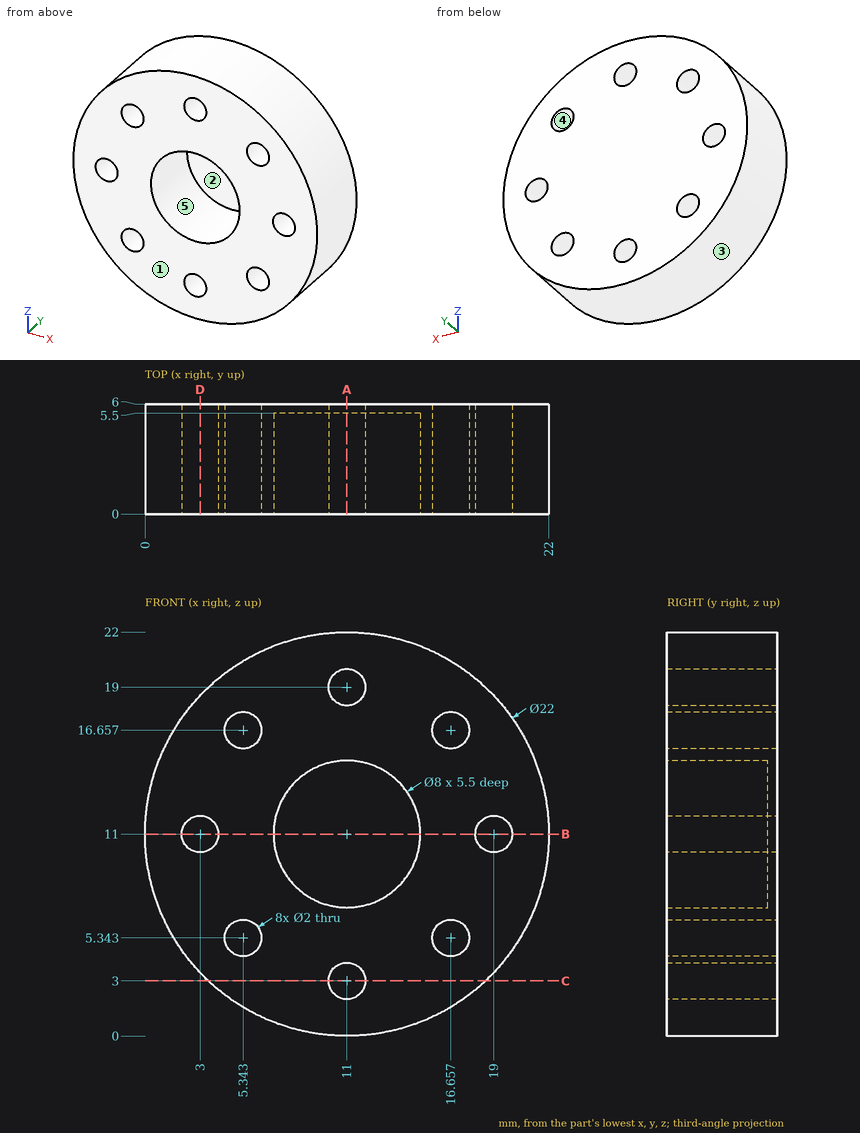
Could you check a few things on this drawing? It's one solid part, dimensions in mm from its lowest x, y, z. A direction names the side the tool comes from. Give positions to 0.01 mm unless a question says otherwise; leave off trailing zeros. Order: outer loops, then holes, each group sorted by start corner. A loop starts at its lowest first (then second) coordinate and runs counter-clockwise, first axis right, second up. Notation, with made-up numbers: (89, -15) - (132, -15) arc R25 cw to (132, 17) - close; hole circle Ø11 at (-8, 71). An arc over 180 degrees is marked (long way). One line per item, written item: value. Start each with the question number.
1. Thinking about a two-plate mould opening in Z: for the marked faces 1, 2 and 3, which applies, +Z half, -Z half, draft (parallel to the pull), parting line (faces both ways), or undercut?
2. Imagine slicing it at C-C on z = 3. List the corners of the cut face in (x, y) for me, plus the area to 3 significant figures.
3. If I drill on probe 1 along X at (y, z) = (5.2, 17.5) (1 decimal); probe 2 along X at (y, z) = (2.9, 10.25) (1 decimal); probe 3 along X at (y, z) = (5.2, 16), over which ranges is the centre line in solid material (lowest first)?
4. Imagine slicing it at B-B on z = 11. List the corners of the cut face in (x, y) for me, plus the area to 3 significant figures.
5. Imagine slicing it at D-D on x = 3. List the corners of the cut face in (y, z) for me.
6. For P1, Ø1.5, axis at y = 2.5, z = 13.5, coming from the -X side; P2, Ø1.5, axis at y = 3, z = 18, coming from the +X side; P3, Ø1.2, axis at x = 3, z = 11, coming from the +Y side; P4, Ø3, axis at x = 17.5, y = 1.5, coming from the -Z side, each with a flat end and sliding along its axis, tell me the tip position at first contact or that it passes through.
7. For the marked faces 4 and 5, which set-ups out of +Z, -Z, +X, -X, +Y, -Y let a thin tool reach every point of the face, with its end or its side?
8. Imagine slicing it at A-A on x = 11. List the corners of the cut face in (y, z) for me.
Values:
1. face 1: draft
1. face 2: undercut
1. face 3: parting line
2. outline: (3.45, 0) - (10, 0) - (10, 6) - (3.45, 6) - close; (12, 0) - (18.55, 0) - (18.55, 6) - (12, 6) - close
2. area: 78.6 mm²
3. probe 1: 2.1 to 4.8, 5.9 to 16.1, 17.2 to 19.9
3. probe 2: 0 to 2.3, 3.7 to 7.1, 14.9 to 18.3, 19.7 to 22
3. probe 3: 1.2 to 4.59, 6.1 to 15.9, 17.41 to 20.8
4. outline: (0, 0) - (2, 0) - (2, 6) - (0, 6) - close; (4, 0) - (7, 0) - (7, 5.5) - (15, 5.5) - (15, 0) - (18, 0) - (18, 6) - (4, 6) - close; (20, 0) - (22, 0) - (22, 6) - (20, 6) - close
4. area: 64.0 mm²
5. outline: (0, 3.45) - (6, 3.45) - (6, 10) - (0, 10) - close; (0, 12) - (6, 12) - (6, 18.55) - (0, 18.55) - close
6. P1: x = 0.14
6. P2: x = 20.05
6. P3: through
6. P4: z = 1.2
7. face 4: +Y, -Y
7. face 5: -Y
8. outline: (0, 0) - (6, 0) - (6, 2) - (0, 2) - close; (0, 4) - (6, 4) - (6, 18) - (0, 18) - (0, 15) - (5.5, 15) - (5.5, 7) - (0, 7) - close; (0, 20) - (6, 20) - (6, 22) - (0, 22) - close
